from build123d import *

# Parameters (mm, degrees)
SKETCH1_W           = 571.5
SKETCH1_H           = 430.53
SKETCH1_W_2         = 469.9
SKETCH1_H_2         = 303.53
BOSS_EXTRUDE1_DEPTH = 15.875
SKETCH2_W           = 240.03
SKETCH2_H           = 15.875
BOSS_EXTRUDE2_DEPTH = 158.75


with BuildPart() as part:
    # Sketch1 → Boss-Extrude1 (new body)
    with BuildSketch(Plane(origin=(0, 0, 0), x_dir=(1, 0, 0), z_dir=(0, 1, 0))):
        with Locations((285.75, 215.265)):
            Rectangle(SKETCH1_W, SKETCH1_H)
        with Locations((285.75, 215.265)):
            Rectangle(SKETCH1_W_2, SKETCH1_H_2, mode=Mode.SUBTRACT)
    extrude(amount=BOSS_EXTRUDE1_DEPTH)

    # Sketch2 → Boss-Extrude2 (add)
    with BuildSketch(Plane.XY):
        with Locations((451.485, 7.9375)):
            Rectangle(SKETCH2_W, SKETCH2_H)
    extrude(amount=BOSS_EXTRUDE2_DEPTH)


solid = part.part
Verification items for the finished model (mm, model axes). A direction names the side the tool comes from. Give positions to 0.01 mm unless a question says otherwise; leave off trailing zeros. Loops run counter-clockwise (first coordinate to the right, second up) from the corner with the lowest first, then second, coordinate; pieces in that order, holes last.
1. Material ranges on probe 1 along Z at (x, y) = (234.5, 12.25); probe 2 along X at (y, z) = (6.25, -147.5); probe 3 along Z at (x, y) = (462, 9.5), recorded low to high.
Derived:
probe 1: z = -430.53 to -367.03, -63.5 to 0
probe 2: x = 0 to 50.8, 520.7 to 571.5
probe 3: z = -430.53 to -367.03, -63.5 to 158.75
2. Cross-section at B-B on z = -235. Record the cut outline in (x, y) (3 decimals), and give its area (3 significant figures).
Derived:
outline: (0, 0) - (50.8, 0) - (50.8, 15.875) - (0, 15.875) - close; (520.7, 0) - (571.5, 0) - (571.5, 15.875) - (520.7, 15.875) - close
area: 1,610 mm2
3. Cross-section at C-C on y = 10. Record the cut outline in (x, z).
Derived:
outline: (0, -430.53) - (571.5, -430.53) - (571.5, 158.75) - (331.47, 158.75) - (331.47, 0) - (0, 0) - close; hole (50.8, -367.03) - (520.7, -367.03) - (520.7, -63.5) - (50.8, -63.5) - close
4. Cross-section at A-A on x = 495. Record the cut outline in (y, z) (3 decimals).
Derived:
outline: (0, -430.53) - (15.875, -430.53) - (15.875, -367.03) - (0, -367.03) - close; (0, -63.5) - (15.875, -63.5) - (15.875, 158.75) - (0, 158.75) - close
5. Release check for a two-part mould opening along Z. For faces 1 (the flat face through (450, 8, 158.75)), 2 (the flat face through (571.5, 8, -140)), 3 (the flat face through (282, 8, -63.5)) record: +Z half, -Z half, draft (parallel to the pull), parting line (faces both ways), or undercut.
Derived:
face 1: +Z half
face 2: draft
face 3: undercut
6. Cross-section at D-D on z = 24. Record the cut outline in (x, y) (3 decimals).
Derived:
outline: (331.47, 0) - (571.5, 0) - (571.5, 15.875) - (331.47, 15.875) - close
7. Tool access check on faces 4 (the flat face through (282, 8, -430.53)), 5 (the flat face through (331.47, 8, 78)), 6 (the flat face through (50.8, 8, -213)). Record the directions out of +Z, -Z, +X, -X, +Y, -Y that give a thin tool (end or side, any length) a straight path to the whole face; none if there is none.
Derived:
face 4: -Z, +X, -X, +Y, -Y
face 5: +Z, -X, +Y, -Y
face 6: +Y, -Y
8. Go/stop test with a flat-tipped pin: P1, Ø8, axis at x = 122, y = 11.5, coming from the +Z side. Record where the tip stops, or that it passes through.
Derived:
P1: stops at z = 0
